```python
from build123d import *

# Parameters (mm, degrees)
FILLET1_R = 0.2
FILLET2_R = 0.2
FILLET3_R = 0.2


with BuildPart() as part:
    # Sketch2 → Revolve1 (revolve)
    with BuildSketch(Plane.XY, mode=Mode.PRIVATE) as revolve1_sk:
        with BuildLine():
            Line((-0.4, -4.75), (-1.638095238, -4.75))
            Line((-1.638095238, -4.75), (-1.638095238, -1.805191747))
            Line((-1.638095238, -1.805191747), (-2.235540304, -1.805191747))
            Line((-2.235540304, -1.805191747), (-2.535540304, 1.194808253))
            Line((-2.535540304, 1.194808253), (-2.093117248, 1.194808253))
            ThreePointArc((-2.093117248, 1.194808253), (-1.879618402, 1.379298482), (-1.8, 1.65))
            Line((-1.8, 1.65), (-1.438630681, 1.65))
            Line((-1.438630681, 1.65), (-1.264172597, 5.25))
            Line((-1.264172597, 5.25), (-0.5, 5.25))
            Line((-0.5, 5.25), (-0.4, 1.65))
            Line((-0.4, 1.65), (-0.4, 1.194808253))
            Line((-0.4, 1.194808253), (-0.4, -1.805191747))
            Line((-0.4, -1.805191747), (-0.4, -4.75))
        make_face()
    revolve(revolve1_sk.sketch.rotate(Axis((0, -5.25, 0), (0, 1, 0)), 270), axis=Axis((0, -5.25, 0), (0, 1, 0)))

    # Fillet1
    fillet1_edges = [part.edges().sort_by_distance(p)[0] for p in [
        (0, 5.25, 1.264172597),
    ]]
    fillet(fillet1_edges, radius=FILLET1_R)

    # Fillet2
    fillet2_edges = [part.edges().sort_by_distance(p)[0] for p in [
        (0, -4.75, 1.638095238),
    ]]
    fillet(fillet2_edges, radius=FILLET2_R)

    # Fillet3
    fillet3_edges = [part.edges().sort_by_distance(p)[0] for p in [
        (0, -1.805191747, 2.235540304),
        (0, 1.194808253, 2.535540304),
    ]]
    fillet(fillet3_edges, radius=FILLET3_R)


solid = part.part
```
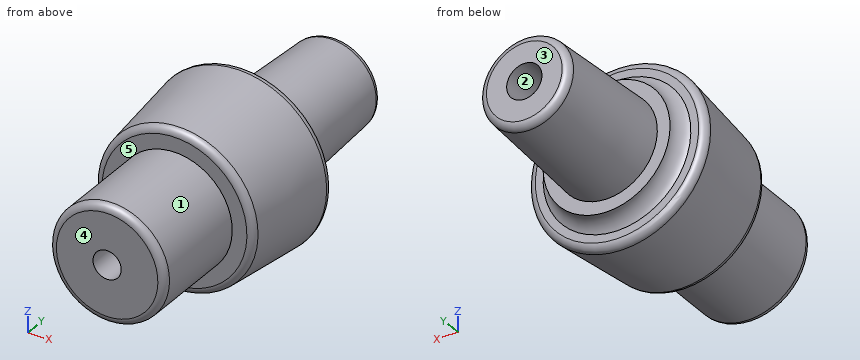
Could you check a few things on this model? Use its own coordinates, in mm. Face numbers are marked on the shaded views. A direction names the side the tool comes from. Coordinates: 2 decimals unless noted, no trailing zeros. Write each loop counter-clockwise with the first axis right and the second up, starting at its lowest first coordinate (ties: lowest second). Pieces come first, ordered by that corner, then holes. Notation, with made-up numbers: (81.25, 6.5) -> (139.25, 6.5) arc R19 ccw to (139.25, 11.5) -> close; hole circle Ø2 at (55.25, -23.75). An arc over 180 degrees is marked (long way). One line per question, with ' | ' between items. Start each with the question number.
1. Thinking about a two-plate mould opening in X: for the marked faces 1, 2 and 3, which applies, pulls with the +X half, pulls with the -X half, needs draft (parallel to the pull), parting line crosses it, or undercut?
2. If we section it at D-D (y = 3.5): Please give me the cut outline in (x, z), and give its area (3 significant figures).
3. Will these pins go through, and if not, where does the flat tip stop? P1, Ø2, axis at x = 1.5, z = 1, coming from the +Y side; P2, Ø2, axis at x = 1.5, y = -3.5, coming from the +Z side.
4. For the marked faces 4 and 5, which set-ups out of +Z, -Z, +X, -X, +Y, -Y let a thin tool reach every point of the face, with its end or its side?
5. If we section it at C-C (y = -4): Please give me the cut outline in (x, z).
6. Please list where these lines run through material, in increasing order: line 1 along X through (y, z) = (-2.5, 0); line 2 along Z through (x, y) = (-0.5, -0.5); line 3 along X through (y, z) = (0.25, 0).
Return value:
1) face 1: parting line crosses it | face 2: undercut | face 3: needs draft
2) outline: circle Ø2.7 at (0, 0); hole circle Ø0.9 at (0, 0) | area: 5.08 mm²
3) P1: stops at y = 5.25 | P2: stops at z = 1.56
4) face 4: +Z, -Z, +X, -X, -Y | face 5: -Y
5) outline: circle Ø3.28 at (0, 0); hole circle Ø0.8 at (0, 0)
6) line 1: x = -1.64 to -0.4, 0.4 to 1.64 | line 2: z = -2.31 to 2.31 | line 3: x = -2.44 to -0.4, 0.4 to 2.44
